from build123d import *

# Parameters (mm, degrees)
ESQUISSE1_R             = 1.5
BOSS_EXTRU_1_DEPTH      = 4.8
ESQUISSE2_R             = 1.7
BOSS_EXTRU_2_DEPTH      = 1.2
BOSS_EXTRU_3_DEPTH      = 0.25
BOSS_EXTRU_3_DEPTH_BACK = 0.25


with BuildPart() as part:
    # Esquisse1 → Boss.-Extru.1 (new body)
    with BuildSketch(Plane(origin=(0, 0, 0), x_dir=(1, 0, 0), z_dir=(0, 1, 0))):
        with Locations(Location((0, 0, 0), (0, 0, 270))):
            Circle(ESQUISSE1_R)
    extrude(amount=-BOSS_EXTRU_1_DEPTH)

    # Esquisse2 → Boss.-Extru.2 (add)
    with BuildSketch(Plane.XZ.offset(4.8)):
        with Locations(Location((0, 0, 0), (0, 0, 270))):
            Circle(ESQUISSE2_R)
    extrude(amount=BOSS_EXTRU_2_DEPTH)

    # Esquisse3 → Boss.-Extru.3 (add, two sides: drawn at the far end of the back side and taken through both)
    with BuildSketch(Plane.XY.offset(-BOSS_EXTRU_3_DEPTH_BACK)):
        with BuildLine():
            Line((0.5, -6), (0.5, -6.672497838))
            Line((0.5, -6.672497838), (0.62, -6.672497838))
            ThreePointArc((0.62, -6.672497838), (0.902842712, -6.789655126), (1.02, -7.072497838))
            Line((1.02, -7.072497838), (1.02, -13.439637098))
            ThreePointArc((1.02, -13.439637098), (-0.163288604, -16.296348494), (-3.02, -17.479637098))
            Line((-3.02, -17.479637098), (-12, -17.479637098))
            Line((-12, -17.479637098), (-12, -17.979637098))
            Line((-12, -17.979637098), (-3.02, -17.979637098))
            ThreePointArc((-3.02, -17.979637098), (0.190264787, -16.649901885), (1.52, -13.439637098))
            Line((1.52, -13.439637098), (1.52, -6.572497838))
            Line((1.52, -6.572497838), (1.084066682, -6))
            Line((1.084066682, -6), (0.5, -6))
        make_face()
        with BuildLine():
            Line((-1.084066682, -6), (-0.5, -6))
            Line((-0.5, -6), (-0.5, -6.672497838))
            Line((-0.5, -6.672497838), (-0.62, -6.672497838))
            ThreePointArc((-0.62, -6.672497838), (-0.902842712, -6.789655126), (-1.02, -7.072497838))
            Line((-1.02, -7.072497838), (-1.02, -13.439637098))
            ThreePointArc((-1.02, -13.439637098), (-1.605786438, -14.85385066), (-3.02, -15.439637098))
            Line((-3.02, -15.439637098), (-12, -15.439637098))
            Line((-12, -15.439637098), (-12, -14.939637098))
            Line((-12, -14.939637098), (-3.02, -14.939637098))
            ThreePointArc((-3.02, -14.939637098), (-1.959339828, -14.50029727), (-1.52, -13.439637098))
            Line((-1.52, -13.439637098), (-1.52, -6.572497838))
            Line((-1.52, -6.572497838), (-1.084066682, -6))
        make_face()
    extrude(amount=BOSS_EXTRU_3_DEPTH + BOSS_EXTRU_3_DEPTH_BACK)


solid = part.part
Geometry: final body of the model. Coordinates: model frame, mm. A direction names the side the tool comes from. Coordinates: 2 decimals unless noted, no trailing zeros. Order: outer loops, then holes, each group sorted by start corner. A loop starts at its lowest first (then second) coordinate and runs counter-clockwise, first axis right, second up. Notation, with made-up numbers: M 84.5,-24 L 143.5,-24 A8 cw 143.5,-9 Z; hole C 13.25,72 d2. An arc over 180 degrees is marked long. One line per question, with ' | ' between items. Start each with the question number.
Item 1: Set-up query: faces 1 (the cylindrical face through (-1.97, -14.51, 0)), 2 (the flat face through (-3.7, -15.2, 0.25)), 3 (the flat face through (-3.7, -15.2, -0.25)). Return all of +Z, -Z, +X, -X, +Y, -Y with unobstructed straight access to the full face (end or side cutting, diameter ignored); none if empty.
Item 2: Cut plane B-B, the plane y = -8.75. Return the cut outline in (x, z), then the cut area to 3 significant figures.
Item 3: Pin query (flat end, axial travel): pin 1 Ø7.5 at (x, y) = (-8, -12.5) entering from -Z; pin 2 Ø0.6 at (y, z) = (-9, 0) entering from +X; pin 3 Ø3 at (x, y) = (0, -3.5) entering from -Z; pin 4 Ø1.7 at (x, z) = (-0.5, 0) entering from -Y. Return the tip coordinate at first contact, or that it passes through.
Item 4: Cut plane D-D, the plane x = 0.25. Return the cut outline in (y, z).
Item 5: Ray query, probe 1 along Y at (x, z) = (-0.5, 0.55); probe 2 along Y at (x, z) = (-1.5, 0.3); probe 3 along X at (y, z) = (-6.25, 0.2). Return the intervals inside material, ascending. Write a range as [from, to].
Item 6: Draft query along Y for faces 4 (the cylindrical face through (-0.13, -16.26, 0)), 5 (the cylindrical face through (0.15, -16.69, 0)), 6 (the flat face through (-1.3, -17.3, 0.25)), 7 (the cylindrical face through (-1.59, -14.84, 0)). Return one class per face: released by +Y, released by -Y, zero draft, split by the parting line, or undercut.
Item 7: Cut plane A-A, the plane x = -11. Return the cut outline in (y, z), then the cut area to 3 significant figures.
A:
1) face 1: +Z, -Z, -X | face 2: +Z, +X, -X, -Y | face 3: -Z, +X, -X, -Y
2) outline: M -1.52,-0.25 L -1.02,-0.25 L -1.02,0.25 L -1.52,0.25 Z; M 1.02,-0.25 L 1.52,-0.25 L 1.52,0.25 L 1.02,0.25 Z | area: 0.500 mm2
3) pin 1: stops at z = -0.25 | pin 2: stops at x = 1.52 | pin 3: stops at z = -1.7 | pin 4: stops at y = -17.66
4) outline: M -16.59,-0.25 L -15.81,-0.25 L -15.81,0.25 L -16.59,0.25 Z; M -6,-1.68 L -4.8,-1.68 L -4.8,-1.48 L 0,-1.48 L 0,1.48 L -4.8,1.48 L -4.8,1.68 L -6,1.68 Z
5) probe 1: y = [-6, 0] | probe 2: y = [-6, -4.8] | probe 3: x = [-1.27, -0.5], [0.5, 1.27]
6) face 4: undercut | face 5: released by -Y | face 6: zero draft | face 7: undercut
7) outline: M -17.98,-0.25 L -17.48,-0.25 L -17.48,0.25 L -17.98,0.25 Z; M -15.44,-0.25 L -14.94,-0.25 L -14.94,0.25 L -15.44,0.25 Z | area: 0.500 mm2
